```python
from build123d import *

# Parameters (mm, degrees)
SKETCH_1_W          = 42
SKETCH_1_H          = 42
SKETCH_1_R          = 1.6
SKETCH_1_R_2        = 12
EXTRUDE_1_DEPTH     = 3
SKETCH_2_W          = 16
SKETCH_2_H          = 52
EXTRUDE_2_DEPTH     = 10
SKETCH_3_R          = 4.1
CUT_EXTRUDE_1_DEPTH = 6
EXTRUDE_3_DEPTH     = 79
SKETCH_7_W          = 16
SKETCH_7_H          = 0.6
CUT_EXTRUDE_4_DEPTH = 49
EXTRUDE_START       = 49.4
EXTRUDE_4_DEPTH     = 26.6
SKETCH_10_W         = 7.1
SKETCH_10_H         = 0.1
SKETCH_10_W_2       = 0.1
SKETCH_10_H_2       = 7.1
CUT_EXTRUDE_5_DEPTH = 76


with BuildPart() as part:
    # 草图1 → 凸台-拉伸1 (new body)
    with BuildSketch(Plane(origin=(0, 0, 0), x_dir=(1, 0, 0), z_dir=(0, 1, 0))):
        Rectangle(SKETCH_1_W, SKETCH_1_H)
        with Locations(Location((15.5, 15.5, 0), (0, 0, 270))):
            Circle(SKETCH_1_R, mode=Mode.SUBTRACT)
        with Locations(Location((15.5, -15.5, 0), (0, 0, 270))):
            Circle(SKETCH_1_R, mode=Mode.SUBTRACT)
        with Locations(Location((-15.5, -15.5, 0), (0, 0, 270))):
            Circle(SKETCH_1_R, mode=Mode.SUBTRACT)
        with Locations(Location((-15.5, 15.5, 0), (0, 0, 270))):
            Circle(SKETCH_1_R, mode=Mode.SUBTRACT)
        with Locations(Location((0, 0, 0), (0, 0, 270))):
            Circle(SKETCH_1_R_2, mode=Mode.SUBTRACT)
    extrude(amount=EXTRUDE_1_DEPTH)

    # 草图2 → 凸台-拉伸2 (add)
    with BuildSketch(Plane.XY.offset(21)):
        with Locations((11, -23)):
            Rectangle(SKETCH_2_W, SKETCH_2_H)
    extrude(amount=EXTRUDE_2_DEPTH)

    # 草图3 → 切除-拉伸1 (cut)
    with BuildSketch(Plane.XY.offset(31)):
        with Locations((11, -29)):
            Circle(SKETCH_3_R)
    extrude(amount=-CUT_EXTRUDE_1_DEPTH, mode=Mode.SUBTRACT)

    # 草图4 → 凸台-拉伸3 (add)
    with BuildSketch(Plane(origin=(0, 3, 0), x_dir=(1, 0, 0), z_dir=(0, 1, 0))):
        Polygon((1, 21), (21, 21), (21, 1), (24, 1), (24, 24), (1, 24), align=None)
    extrude(amount=-EXTRUDE_3_DEPTH)

    # 草图7 → 切除-拉伸4 (cut)
    with BuildSketch(Plane.XZ.offset(49)):
        with Locations((11, 21.3)):
            Rectangle(SKETCH_7_W, SKETCH_7_H)
    extrude(amount=-CUT_EXTRUDE_4_DEPTH, mode=Mode.SUBTRACT)

    # 草图9 → 凸台-拉伸4 (add)
    with BuildSketch(Plane.XZ.offset(EXTRUDE_START)):
        Polygon((8.33, -15.1), (13.667157288, -15.1), (16.3, -17.732842712), (16.3, -19.3), (13.9, -19.3), (13.9, -21), (8.1, -21), (8.1, -19.3), (5.7, -19.3), (5.7, -17.73), align=None)
    extrude_4 = extrude(amount=EXTRUDE_4_DEPTH)

    # 镜向1: 凸台-拉伸4 across plane
    add(extrude_4.mirror(Plane(origin=(0, 0, 0), x_dir=(-0.7071067811865475, 0, 0.7071067811865476), z_dir=(-0.7071067811865478, 0, -0.7071067811865474))))

    # 草图10 → 切除-拉伸5 (cut)
    with BuildSketch(Plane.XZ.offset(76)):
        with Locations((4.55, -21.05)):
            Rectangle(SKETCH_10_W, SKETCH_10_H)
        with Locations((17.45, -21.05)):
            Rectangle(SKETCH_10_W, SKETCH_10_H)
        with Locations((21.05, -21.05)):
            Rectangle(SKETCH_10_W_2, SKETCH_10_H)
        with Locations((21.05, -17.45)):
            Rectangle(SKETCH_10_W_2, SKETCH_10_H_2)
    extrude(amount=-CUT_EXTRUDE_5_DEPTH, mode=Mode.SUBTRACT)


solid = part.part
```
Verification items for the finished model (mm, model axes). A direction names the side the tool comes from. Give positions to 0.01 mm unless a question says otherwise; leave off trailing zeros. Order: outer loops, then holes, each group sorted by start corner. A loop starts at its lowest first (then second) coordinate and runs counter-clockwise, first axis right, second up. Notation, with made-up numbers: (-23.75, 17.5) -> (21.25, 17.5) arc R22 cw to (21.25, 34.5) -> close; hole circle Ø1 at (50, 64.5). An arc over 180 degrees is marked (long way). One line per item, written item: value.
(1) Sectioned sample at D-D on z = 9.5. Record the cut outline in (x, y), then the cut area to 3 significant figures.
Final values:
outline: (-21, 0) -> (-7.33, 0) -> (-7.33, 3) -> (-21, 3) -> close; (7.33, 0) -> (21, 0) -> (21, 3) -> (7.33, 3) -> close
area: 82.0 mm^2
(2) Scan lines: line 1 along X through (y, z) = (1, -15.5); line 2 along X through (y, z) = (1.25, 15.5); line 3 along Z through (x, y) = (-15, 1). Record each from-to range of solid material in increasing order. Write a range as [from, to].
Final values:
line 1: [-21, -17.1], [-13.9, 13.9], [17.1, 24]
line 2: [-21, -17.1], [-13.9, 13.9], [17.1, 21]
line 3: [-21, -17.02], [-13.98, 13.98], [17.02, 21]
(3) Sectioned sample at A-A on y = -29. Record the cut outline in (x, z), then the cut area to 3 significant figures.
Final values:
outline: (1, -24) -> (24, -24) -> (24, -1) -> (21, -1) -> (21, -13.9) -> (21.1, -13.9) -> (21.1, -21.1) -> (13.9, -21.1) -> (13.9, -21) -> (8.1, -21) -> (8.1, -21.1) -> (1, -21.1) -> close; (3, 21.6) -> (19, 21.6) -> (19, 31) -> (15.1, 31) -> (15.1, 25) -> (6.9, 25) -> (6.9, 31) -> (3, 31) -> close
area: 228 mm^2
(4) Tool access check on faces 5 (the face through (11, -63, -15.1)), 6 (the face through (21, 1, 10)), 7 (the face through (14.965, -62.514, -16.398)). Record the directions out of +Z, -Z, +X, -X, +Y, -Y that give a thin tool (end or side, any length) a straight path to the whole face; none if there is none.
Final values:
face 5: +Z, -X, -Y
face 6: +Z, +X, +Y, -Y
face 7: -Y
(5) Gauge pin test, flat ends, axial feed: pin 1 (8 mm diameter, centred on x = 3, z = 22.5, fed in from -Y); pin 2 (1 mm diameter, centred on y = -21.5, z = -11.5, fed in from -X); pin 3 (10 mm diameter, centred on y = -48.5, z = 5.5, fed in from -X); pin 4 (10.5 mm diameter, centred on x = 11, y = -29, fed in from +Z). Record the tip position at first contact, or that the pin passes through.
Final values:
pin 1: y = -49
pin 2: x = 21
pin 3: through
pin 4: z = 31
(6) Sectioned sample at B-B on z = 15.5. Record the cut outline in (x, y).
Final values:
outline: (-21, 0) -> (-17.1, 0) -> (-17.1, 3) -> (-21, 3) -> close; (-13.9, 0) -> (13.9, 0) -> (13.9, 3) -> (-13.9, 3) -> close; (17.1, 0) -> (21, 0) -> (21, 3) -> (17.1, 3) -> close
(7) Draft check along Z on faces 1 (the face through (19.3, -63, -15)), 2 (the face through (22, -36, -1)), 3 (the face through (1, -36, -23)), 4 (the face through (11, -25, 21.6)). Enter one of: pulls with the +Z half, pulls with the -Z half, needs draft (parallel to the pull), parting line crosses it, or undercut.
Final values:
face 1: undercut
face 2: pulls with the +Z half
face 3: needs draft
face 4: undercut
(8) Sectioned sample at C-C on x = 4. Record the cut outline in (y, z), then the cut area to 3 significant figures.
Final values:
outline: (-76, -24) -> (3, -24) -> (3, -11.31) -> (0, -11.31) -> (0, -21.1) -> (-76, -21.1) -> close; (-49, 21.6) -> (0, 21.6) -> (0, 11.31) -> (3, 11.31) -> (3, 31) -> (-49, 31) -> close
area: 778 mm^2
